from build123d import *

# Parameters (mm, degrees)
BOSS_EXTRUDE1_DEPTH = 0.254
SKETCH2_R           = 4.699
CUT_EXTRUDE1_DEPTH  = 1.254
SKETCH3_W           = 2.54
SKETCH3_H           = 0.635
CUT_EXTRUDE2_DEPTH  = 1.254
SKETCH5_OUTSIDE_W   = 121.447
SKETCH5_OUTSIDE_H   = 109.618
CUT_EXTRUDE5_DEPTH  = 1.254


with BuildPart() as part:
    # Sketch1 → Boss-Extrude1 (new body)
    with BuildSketch(Plane.XY):
        with BuildLine():
            Line((67.21146711, 76.191723231), (8.696654013, 17.676910134))
            Line((8.696654013, 17.676910134), (7.228954972, 14.133571205))
            ThreePointArc((7.228954972, 14.133571205), (14.666587579, 6.075099489), (15.105587123, -4.88230096))
            Line((15.105587123, -4.88230096), (18.648926052, -6.35))
            Line((18.648926052, -6.35), (101.401368334, -6.35))
            ThreePointArc((101.401368334, -6.35), (93.866160503, 38.880636728), (67.21146711, 76.191723231))
        make_face()
        with BuildLine():
            Line((88.672924278, 6.35), (27.86051193, 6.35))
            ThreePointArc((27.86051193, 6.35), (26.399857642, 10.93517908), (24.190484974, 15.210228852))
            Line((24.190484974, 15.210228852), (67.191354125, 58.211098004))
            ThreePointArc((67.191354125, 58.211098004), (82.13289044, 34.020557137), (88.672924278, 6.35))
        make_face(mode=Mode.SUBTRACT)
    extrude(amount=BOSS_EXTRUDE1_DEPTH)

    # Sketch2 → Cut-Extrude1 (cut, through all)
    with BuildSketch(Plane.XY.offset(0.254)):
        with Locations((22.225, 0)):
            Circle(SKETCH2_R)
        with Locations((36.195, 0)):
            Circle(SKETCH2_R)
        with Locations((61.722, 0)):
            Circle(SKETCH2_R)
        with Locations((75.692, 0)):
            Circle(SKETCH2_R)
        with Locations((95.25, 0)):
            Circle(SKETCH2_R)
        with Locations((15.715448212, 15.715448212)):
            Circle(SKETCH2_R)
        with Locations((25.593729945, 25.593729945)):
            Circle(SKETCH2_R)
        with Locations((43.644044748, 43.644044748)):
            Circle(SKETCH2_R)
        with Locations((53.522326482, 53.522326482)):
            Circle(SKETCH2_R)
        with Locations((92.004434954, 24.652514046)):
            Circle(SKETCH2_R)
        with Locations((82.48891971, 47.625)):
            Circle(SKETCH2_R)
        with Locations((67.351920908, 67.351920908)):
            Circle(SKETCH2_R)
    extrude(amount=-CUT_EXTRUDE1_DEPTH, mode=Mode.SUBTRACT)

    # Sketch3 → Cut-Extrude2 (cut, through all)
    with BuildSketch(Plane.XY.offset(0.254)):
        Polygon((15.266435406, 24.246691527), (17.06248663, 26.042742751), (17.511499436, 25.593729945), (15.715448212, 23.797678721), align=None)
        Polygon((44.991083167, 53.971339288), (43.195031942, 52.175288063), (43.644044748, 51.726275257), (45.440095973, 53.522326482), align=None)
        with Locations((29.21, -6.0325)):
            Rectangle(SKETCH3_W, SKETCH3_H)
        with Locations((68.707, -6.0325)):
            Rectangle(SKETCH3_W, SKETCH3_H)
        Polygon((29.230733674, 38.210989795), (31.026784898, 40.007041019), (31.475797704, 39.558028213), (29.67974648, 37.761976989), align=None)
        Polygon((56.845021246, 65.825277367), (55.048970022, 64.029226143), (55.497982828, 63.580213337), (57.294034052, 65.376264561), align=None)
        with Locations((48.9585, -6.0325)):
            Rectangle(SKETCH3_W, SKETCH3_H)
        with Locations((85.471, -6.0325)):
            Rectangle(SKETCH3_W, SKETCH3_H)
        Polygon((99.935462164, 14.437711971), (100.266998693, 11.919442024), (101.526133667, 12.085210288), (101.194597138, 14.603480236), align=None)
        Polygon((93.765504959, 37.464305742), (94.938831965, 37.950313702), (93.966816047, 40.296967714), (92.793489041, 39.810959755), align=None)
        Polygon((79.327792988, 62.471156422), (80.874047017, 60.456038938), (81.88160576, 61.229165953), (80.33535173, 63.244283437), align=None)
        Polygon((13.593916116, 7.005422516), (14.565932035, 4.658768503), (15.739259041, 5.144776462), (14.767243123, 7.491430475), align=None)
    extrude(amount=-CUT_EXTRUDE2_DEPTH, mode=Mode.SUBTRACT)

    # Sketch5 outside → Cut-Extrude5 (cut, through all)
    with BuildSketch(Plane.XY.offset(0.254)):
        with Locations((54.4145, 34.921)):
            Rectangle(SKETCH5_OUTSIDE_W, SKETCH5_OUTSIDE_H)
        with BuildLine():
            Line((81.437068577, 32.35770019), (95.518252433, 38.190317518))
            ThreePointArc((95.518252433, 38.190317518), (99.36478975, 26.62471517), (101.816391891, 14.685341068))
            Line((101.816391891, 14.685341068), (86.705420292, 12.695943916))
            ThreePointArc((86.705420292, 12.695943916), (84.644080158, 22.680312922), (81.437068577, 32.35770019))
        make_face(mode=Mode.SUBTRACT)
    extrude(amount=-CUT_EXTRUDE5_DEPTH, mode=Mode.SUBTRACT)


solid = part.part
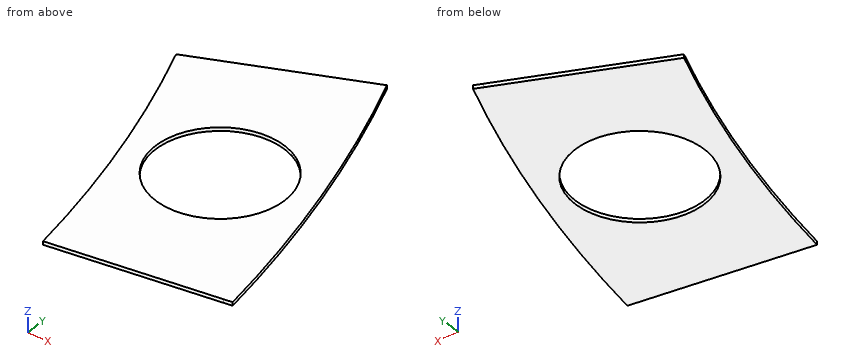
Build history of the part. All positions in model axes, mm. Coordinates: 2 decimals unless noted, no trailing zeros. Order: outer loops, then holes, each group sorted by start corner. A loop starts at its lowest first (then second) coordinate and runs counter-clockwise, first axis right, second up. Notation, with made-up numbers: M 6,45 L 18,45 A5 ccw 18,51 Z; hole C -26,-35.75 d7. An arc over 180 degrees is marked long. One line per question, with ' | ' between items. Start each with the question number.
Q1. Saw through at B-B (y = 22). List the corners of the cut face in (x, z).
Q2. Saw through at C-C (z = 0.2). List the corners of the cut face in (x, y).
Q3. Saw through at A-A (x = 91.25). List the corners of the cut face in (y, z), then the cut area to 3 significant figures.
Q4. Probe L1, parallel to Y at x = 94, z = 0.1; L2, parallel to Y at x = 89, z = 0.2; L3, parallel to X at y = 26, z = 0.1. List the from-to ranges inside material, lowest first. Write a range as from..to.
Q5. Flat gauge pin, fed straight in: pin 1 Ø8 at (x, y) = (86, 19) entering from -Z. Where does the tip first touch, or does it go through?
Q6. Saw through at D-D (y = 17). List the corners of the cut face in (x, z), then the cut area to 3 significant figures.
Check values:
1) outline: M 86.13,0 L 88.13,0 L 88.13,0.25 L 86.13,0.25 Z; M 95.88,0 L 99.19,0 L 99.19,0.25 L 95.88,0.25 Z
2) outline: M 82.61,32.84 A88.9 cw 87.96,12.86 L 100.56,14.52 A101.6 ccw 94.34,37.7 Z; hole C 92,24.65 d9.4
3) outline: M 13.29,0 L 20.01,0 L 20.01,0.25 L 13.29,0.25 Z; M 29.29,0 L 36.42,0 L 36.42,0.25 L 29.29,0.25 Z | area: 3.52 mm2
4) L1: y = 13.66..20.4, 28.91..37.56 | L2: y = 13..21.04, 28.27..35.49 | L3: x = 85.01..87.5, 96.51..98.22
5) pin 1: stops at z = 0
6) outline: M 87.26,0 L 100.17,0 L 100.17,0.25 L 87.26,0.25 Z | area: 3.28 mm2
